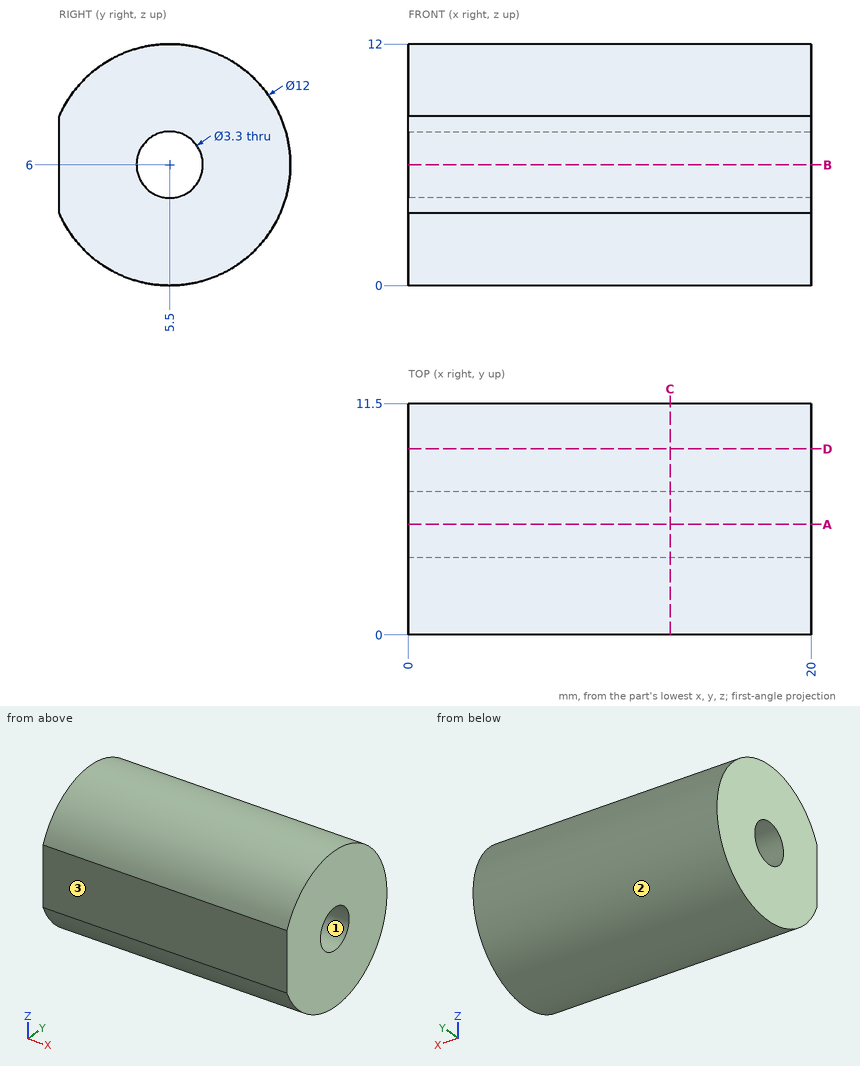
Could you check a few things on this drawing? It's one solid part, dimensions in mm from its lowest x, y, z. Round coordinates to 2 decimals unless told otherwise and drop trailing zeros. Order: outer loops, then holes, each group sorted by start corner. A loop starts at its lowest first (then second) coordinate and runs counter-clockwise, first axis right, second up. Notation, with made-up numbers: M 0,57 L 49,57 A13 cw 49,72 Z; hole C -40,57 d9. An arc over 180 degrees is marked long. One line per question, with ' | ' between items. Start each with the question number.
(1) Suppose I cut it at C-C on x = 13. List the corners of the cut face in (y, z) for me.
(2) Thinking about a two-plate mould opening in Z: for the marked faces 1, 2 and 3, which applies, +Z half, -Z half, draft (parallel to the pull), parting line (faces both ways), or undercut?
(3) Suppose I cut it at A-A on y = 5.5. List the corners of the cut face in (x, z) for me.
(4) Please list where these lines run through material, in increasing order: line 1 along Y through (x, z) = (14.75, 6); line 2 along Z through (x, y) = (10.25, 4); line 3 along Z through (x, y) = (3.25, 6.75).
(5) Suppose I cut it at B-B on z = 6. List the corners of the cut face in (x, y) for me, then the cut area to 3 significant figures.
(6) Suppose I cut it at D-D on y = 9.25. List the corners of the cut face in (x, z) for me, then the cut area to 3 significant figures.
(7) For P1, Ø2, axis at x = 15, y = 7, coming from the -Z side; P2, Ø1.5, axis at y = 5, z = 9, coming from the -X side, each with a flat end and sliding along its axis, tell me the tip position at first contact or that it passes through.
Geometry results:
1) outline: M 0,3.6 A6 ccw long 0,8.4 Z; hole C 5.5,6 d3.3
2) face 1: undercut | face 2: parting line | face 3: draft
3) outline: M 0,0 L 20,0 L 20,4.35 L 0,4.35 Z; M 0,7.65 L 20,7.65 L 20,12 L 0,12 Z
4) line 1: 0 to 3.85, 7.15 to 11.5 | line 2: 0.19 to 5.31, 6.69 to 11.81 | line 3: 0.13 to 4.92, 7.08 to 11.87
5) outline: M 0,0 L 20,0 L 20,3.85 L 0,3.85 Z; M 0,7.15 L 20,7.15 L 20,11.5 L 0,11.5 Z | area: 164 mm²
6) outline: M 0,1.32 L 20,1.32 L 20,10.68 L 0,10.68 Z | area: 187 mm²
7) P1: z = 0.02 | P2: x = 0
